Source: CAD feature listing. Evaluate the final solid. Frame: model axes, mm. A direction names the side the tool comes from. Round coordinates to 2 decimals unless told otherwise and drop trailing zeros. Write each loop counter-clockwise with the first axis right and the second up, starting at its lowest first coordinate (ties: lowest second). Pieces come first, ordered by that corner, then holes. Notation, with made-up numbers: M -12,-4.75 L 41,-4.75 A16 ccw 41,2.25 Z; hole C 30.25,28.5 d3. An arc over 180 degrees is marked long. Use a Markdown table: item, result.
```python
from build123d import *

# Parameters (mm, degrees)
BOSS_EXTRUDE1_DEPTH       = 28.321
SKETCH2_R                 = 4.7625
BOSS_EXTRUDE2_DEPTH       = 6.35
SKETCH3_R                 = 6.35
BOSS_EXTRUDE3_DEPTH       = 38.1
F_8_32_TAPPED_HOLE1_D     = 3.4544
F_8_32_TAPPED_HOLE1_DEPTH = 10.668
F_8_32_TAPPED_HOLE1_TIP   = 1.037806461
SKETCH7_R                 = 3.175
CUT_EXTRUDE2_DEPTH        = 6.35


with BuildPart() as part:
    # Sketch1 → Boss-Extrude1 (new body)
    with BuildSketch(Plane(origin=(0, 0, 0), x_dir=(1, 0, 0), z_dir=(0, 1, 0))):
        Polygon((6.35, -3.666174209), (6.35, 3.666174209), (0, 7.332348419), (-6.35, 3.666174209), (-6.35, -3.666174209), (0, -7.332348419), align=None)
    extrude(amount=BOSS_EXTRUDE1_DEPTH)

    # Sketch2 → Boss-Extrude2 (add)
    with BuildSketch(Plane.XZ):
        Circle(SKETCH2_R)
    extrude(amount=BOSS_EXTRUDE2_DEPTH)

    # Sketch3 → Boss-Extrude3 (add)
    with BuildSketch(Plane(origin=(0, 28.321, 0), x_dir=(1, 0, 0), z_dir=(0, 1, 0))):
        Circle(SKETCH3_R)
    extrude(amount=BOSS_EXTRUDE3_DEPTH)

    # #8-32 Tapped Hole1
    with Locations(Plane(origin=(0, 66.421, 0), x_dir=(1, 0, 0), z_dir=(0, 1, 0))):
        with Locations((0, 0)):
            Hole(F_8_32_TAPPED_HOLE1_D / 2, depth=F_8_32_TAPPED_HOLE1_DEPTH)
            with Locations((0, 0, -(F_8_32_TAPPED_HOLE1_DEPTH + F_8_32_TAPPED_HOLE1_TIP / 2))):  # 118° drill point
                Cone(0, F_8_32_TAPPED_HOLE1_D / 2, F_8_32_TAPPED_HOLE1_TIP, mode=Mode.SUBTRACT)

    # Sketch7 → Cut-Extrude2 (cut)
    with BuildSketch(Plane.XZ.offset(6.35)):
        Circle(SKETCH7_R)
    extrude(amount=-CUT_EXTRUDE2_DEPTH, mode=Mode.SUBTRACT)


solid = part.part
```
Q1. Section B-B on y = 61.5. Return loops of the section in (x, z), plus the area to 3 significant figures.
Results are:
| item | result |
|---|---|
| outline | C 0,0 d12.7; hole C 0,0 d3.45 |
| area | 117 mm^2 |
Q2. Mould query, pull axis Z, two halves, no side actions, for faces 4 (the conical face through (0.14, 54.9, 0.27)), 5 (the flat face through (3.219, 13.962, -5.474)), 6 (the flat face through (3.131, 13.962, 5.525)). Classes: +Z half, -Z half, draft (parallel to the pull), parting line (faces both ways), or undercut.
Results are:
| item | result |
|---|---|
| face 4 | undercut |
| face 5 | -Z half |
| face 6 | +Z half |
Q3. Section C-C on y = 40.5. Return loops of the section in (x, z), plus the area to 3 significant figures.
Results are:
| item | result |
|---|---|
| outline | C 0,0 d12.7 |
| area | 127 mm^2 |
Q4. Line query: L1, parallel to Z at x = 0, y = 64; L2, parallel to Y at x = 0, z = 6; L3, parallel to Z at x = -0.25, y = 49.5. Output: solid intervals per line, ascending.
Results are:
| item | result |
|---|---|
| L1 | -6.35 to -1.73, 1.73 to 6.35 |
| L2 | 0 to 66.42 |
| L3 | -6.35 to 6.35 |
Q5. Section A-A on y = 6.5. Return loops of the section in (x, z).
Results are:
| item | result |
|---|---|
| outline | M -6.35,-3.67 L 0,-7.33 L 6.35,-3.67 L 6.35,3.67 L 0,7.33 L -6.35,3.67 Z |
Q6. First-contact query: pin 1 Ø5 at (x, y) = (0.5, 22) entering from -Z; pin 2 Ø4 at (x, z) = (0, 0) entering from -Y; pin 3 Ø1.5 at (x, y) = (-0.5, 55.5) entering from -Z. Flat tips, straight axial feed; report the tip coordinate or a pass-through.
Results are:
| item | result |
|---|---|
| pin 1 | z = -7.33 |
| pin 2 | y = 0 |
| pin 3 | z = -6.35 |
Q7. Reachability of faces 1 (the flat face through (0, 0, 0)), 2 (the flat face through (0, 28.321, 7)), 3 (the flat face through (-6, 28.321, 3)) from +Z, -Z, +X, -X, +Y, -Y: full face, straight path, thin tool, end or side. Return the list, or none.
Results are:
| item | result |
|---|---|
| face 1 | -Y |
| face 2 | +Z, +Y |
| face 3 | +Z, -X, +Y |
